Verification items for the finished model (mm, model axes). Round coordinates to 2 decimals unless told otherwise and drop trailing zeros. Order: outer loops, then holes, each group sorted by start corner. A loop starts at its lowest first (then second) coordinate and runs counter-clockwise, first axis right, second up. Notation, with made-up numbers: (-11, 46.5) -> (0, 46.5) arc R6 cw to (0, 57.5) -> close; hole circle Ø2 at (77.5, 69). An arc over 180 degrees is marked (long way). Put each result on its own line as item: value.
from build123d import *

# Parameters (mm, degrees)
SZKIC1_R                    = 3
SZKIC1_R_2                  = 3.5
DODANIE_WYCI_GNI_CIE1_DEPTH = 5


with BuildPart() as part:
    # Szkic1 → Dodanie-wyciągnięcie1 (new body)
    with BuildSketch(Plane.XY):
        with BuildLine():
            Line((-6, -40), (-6, 0))
            ThreePointArc((-6, 0), (0, 6), (6, 0))
            Line((6, 0), (6, -40))
            ThreePointArc((6, -40), (0, -46), (-6, -40))
        make_face()
        Circle(SZKIC1_R, mode=Mode.SUBTRACT)
        with Locations((0, -40)):
            Circle(SZKIC1_R_2, mode=Mode.SUBTRACT)
    extrude(amount=DODANIE_WYCI_GNI_CIE1_DEPTH)


solid = part.part
Item 1: Material ranges on L1, parallel to Y at x = 0, z = 3.85; L2, parallel to Y at x = -2.5, z = 4; L3, parallel to X at y = -43, z = 0.85, recorded low to high. Write a range as [from, to].
Check sheet entries:
L1: y = [-46, -43.5], [-36.5, -3], [3, 6]
L2: y = [-45.45, -42.45], [-37.55, -1.66], [1.66, 5.45]
L3: x = [-5.2, -1.8], [1.8, 5.2]
Item 2: Section check D-D on x = -2.5. Record the boundary of the cut face in (y, z).
Check sheet entries:
outline: (-45.45, 0) -> (-42.45, 0) -> (-42.45, 5) -> (-45.45, 5) -> close; (-37.55, 0) -> (-1.66, 0) -> (-1.66, 5) -> (-37.55, 5) -> close; (1.66, 0) -> (5.45, 0) -> (5.45, 5) -> (1.66, 5) -> close
Item 3: Release check for a two-part mould opening along X. For faces 1 (the flat face through (-6, -20, 2)), 2 (the cylindrical face through (-0.46, -36.53, 2.46)), 3 (the flat face through (0, -20, 0)), 4 (the cylindrical face through (0, -46, 2)) record: +X half, -X half, draft (parallel to the pull), parting line (faces both ways), or undercut.
Check sheet entries:
face 1: -X half
face 2: undercut
face 3: draft
face 4: parting line
Item 4: Gauge pin test, flat ends, axial feed: pin 1 Ø1 at (x, z) = (1.5, 2) entering from +Y; pin 2 Ø3.5 at (x, y) = (0, 0) entering from +Z. Record the tip position at first contact, or that the pin passes through.
Check sheet entries:
pin 1: stops at y = 5.92
pin 2: passes through
Item 5: Section check C-C on y = -38. Record the boundary of the cut face in (x, z), then the cut area to 3 significant figures.
Check sheet entries:
outline: (-6, 0) -> (-2.87, 0) -> (-2.87, 5) -> (-6, 5) -> close; (2.87, 0) -> (6, 0) -> (6, 5) -> (2.87, 5) -> close
area: 31.3 mm^2
Item 6: Section check B-B on z = 2.9. Record the boundary of the cut face in (x, y), then the cut area to 3 significant figures.
Check sheet entries:
outline: (-6, -40) arc R6 ccw to (6, -40) -> (6, 0) arc R6 ccw to (-6, 0) -> close; hole circle Ø7 at (0, -40); hole circle Ø6 at (0, 0)
area: 526 mm^2
Item 7: Section check A-A on x = 0. Record the boundary of the cut face in (y, z).
Check sheet entries:
outline: (-46, 0) -> (-43.5, 0) -> (-43.5, 5) -> (-46, 5) -> close; (-36.5, 0) -> (-3, 0) -> (-3, 5) -> (-36.5, 5) -> close; (3, 0) -> (6, 0) -> (6, 5) -> (3, 5) -> close
